Design review of the part built by this model. Coordinates are the model's own, in mm. Face numbers are marked on the shaded views. A direction names the side the tool comes from. Round coordinates to 2 decimals unless told otherwise and drop trailing zeros. Write each loop counter-clockwise with the first axis right and the second up, starting at its lowest first coordinate (ties: lowest second). Pieces come first, ordered by that corner, then holes. Notation, with made-up numbers: M 85.25,63.25 L 129.25,63.25 A18 cw 129.25,91.25 Z; hole C -22,88.5 d4. An arc over 180 degrees is marked long. One line per question, with ' | ' between items. Start each with the question number.
Item 1: Add section C-C, the plane y = 33. State the section outline as (x, z) points.
Item 2: Insertion check: pin 1 Ø4 at (x, y) = (34, 14.5) entering from -Z; pin 2 Ø1 at (y, z) = (25.5, 4.5) entering from +X; pin 3 Ø3 at (x, z) = (6, 17.5) entering from -Y. Each pin has a flat end and moves straight along its axis. Give the tip position at first contact, or say it passes through.
Item 3: Draft analysis for pull direction X (two halves, no side actions). For the marked faces 5, 6 and 7, state which applies: released by +X, released by -X, zero draft, split by the parting line, or undercut.
Item 4: Add section B-B, the plane x = 17. State the section outline as (y, z) points, and give its area (3 significant figures).
Item 5: Add section A-A, the plane z = 14.75. State the section outline as (x, y) points, and give its area (3 significant figures).
Item 6: Add section D-D, the plane z = 1. State the section outline as (x, y) points, and give its area (3 significant figures).
Item 7: For L1, parallel to Z at x = 20, y = 34.5; L2, parallel to X at y = 32.5, z = 22.25; L3, parallel to Z at x = 35, y = 28, list the stretches that pass through material, from the lowest coordinate up.
Item 8: Machinability: for the marked faces 1, 2, 3 and 4, which of the approach directions +Z, -Z, +X, -X, +Y, -Y give a long, thin tool a straight path to every point of the face, cutting with its end or side? Answer none if there is none.
```python
from build123d import *

# Parameters (mm, degrees)
SKETCH_W        = 100
SKETCH_H        = 140
PAD_DEPTH       = 2
PAD001_DEPTH    = 22
POCKET_DEPTH    = 2.5
POCKET001_DEPTH = 19.5
POCKET002_DEPTH = 2.001
SKETCH005_R     = 3
PAD002_DEPTH    = 2
SKETCH006_W     = 13
SKETCH006_H     = 5
POCKET003_DEPTH = 50.8979696197


with BuildPart() as part:
    # Sketch → Pad (new body)
    with BuildSketch(Plane.XY):
        with Locations((50, 70)):
            Rectangle(SKETCH_W, SKETCH_H)
    extrude(amount=PAD_DEPTH)

    # Sketch001 (on Face6 of Pad) → Pad001 (join)
    with BuildSketch(Plane.XY.offset(2)):
        Polygon((3, 15.0208152802), (29.162950904, 41.1837661841), (41.1837661842, 29.1629509039), (15.0208152802, 3), align=None)
    extrude(amount=PAD001_DEPTH)

    # Sketch002 (on Face11 of Pad001) → Pocket (cut)
    with BuildSketch(Plane.XY.offset(24)):
        Polygon((5.8284271247, 15.0208152802), (29.162950904, 38.3553390594), (38.3553390594, 29.1629509039), (15.0208152802, 5.8284271247), align=None)
    extrude(amount=-POCKET_DEPTH, mode=Mode.SUBTRACT)

    # Sketch003 (on Face16 of Pocket) → Pocket001 (cut)
    with BuildSketch(Plane.XY.offset(21.5)):
        Polygon((9.3639610307, 18.5563491861), (25.627416998, 34.8198051534), (34.8198051534, 25.6274169979), (18.5563491861, 9.3639610307), align=None)
    extrude(amount=-POCKET001_DEPTH, mode=Mode.SUBTRACT)

    # Sketch004 (on Face5 of Pocket001) → Pocket002 (cut, through all)
    with BuildSketch(Plane.XY.offset(2)):
        Polygon((-2.5188567426, 20.5396720228), (19.697648952, -1.6768336718), (-2.5188567426, -1.6768336718), align=None)
        Polygon((-7.257704, 45), (25.3467170881, 45), (45, 25.3467170881), (45, -9.128844), (123.673981, -9.128844), (123.673981, 160.15947), (-17.63995, 152.949585), align=None)
    extrude(amount=-POCKET002_DEPTH, mode=Mode.SUBTRACT)

    # Sketch005 (on Face2 of Pocket002) → Pad002 (join)
    with BuildSketch(Plane(origin=(0, 0, 0), x_dir=(1, 0, 0), z_dir=(0, 0, -1))):
        with Locations((18.1320851174, -18.1320851174)):
            Circle(SKETCH005_R)
    extrude(amount=PAD002_DEPTH)

    # Sketch006 (on Face11 of Pad002) → Pocket003 (cut, through all)
    with BuildSketch(Plane(origin=(9.0104076401, 9.0104076401, 0), x_dir=(0.7071067812, -0.7071067812, 0), z_dir=(-0.7071067812, -0.7071067812, 0))):
        with Locations((0, 4.5)):
            Rectangle(SKETCH006_W, SKETCH006_H)
    extrude(amount=-POCKET003_DEPTH, mode=Mode.SUBTRACT)


solid = part.part
```
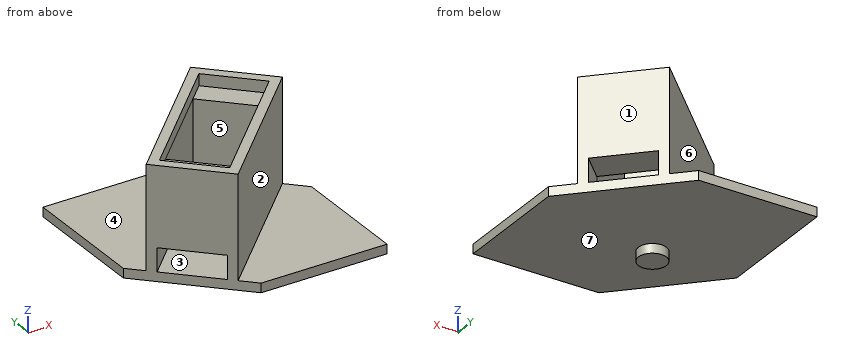
Computed values:
1) outline: M 0,0 L 37.35,0 L 37.35,2 L 23.81,2 L 23.81,24 L 20.98,24 L 20.98,2 L 0,2 Z; M 27.45,7 L 37.35,7 L 37.35,24 L 34.52,24 L 34.52,21.5 L 27.45,21.5 Z
2) pin 1: stops at z = 0 | pin 2: stops at x = 38.02 | pin 3: stops at y = 10.52
3) face 5: undercut | face 6: released by -X | face 7: zero draft
4) outline: M 1.02,0 L 15.35,0 L 15.35,-2 L 20.91,-2 L 20.91,0 L 45,0 L 45,2 L 29.02,2 L 29.02,24 L 26.19,24 L 26.19,2 L 7.81,2 L 7.81,7 L 10.92,7 L 10.92,21.5 L 7.81,21.5 L 7.81,24 L 4.98,24 L 4.98,2 L 1.02,2 Z | area: 269 mm^2
5) outline: M 3,15.02 L 15.02,3 L 41.18,29.16 L 29.16,41.18 Z; hole M 9.36,18.56 L 18.56,9.36 L 34.82,25.63 L 25.63,34.82 Z | area: 330 mm^2
6) outline: M 0,18.02 L 18.02,0 L 45,0 L 45,25.35 L 25.35,45 L 0,45 Z | area: 1,670 mm^2
7) L1: z = 0 to 2 | L2: x = 20.48 to 23.31, 35.02 to 37.85 | L3: z = 0 to 2, 7 to 21.5
8) face 1: +Z, -Z, +X, +Y | face 2: +Z, +X, -Y | face 3: none | face 4: +Z, -X, +Y
